Build history of the part. All positions in model axes, mm. Face numbers are marked on the shaded views. Round coordinates to 2 decimals unless told otherwise and drop trailing zeros. Write each loop counter-clockwise with the first axis right and the second up, starting at its lowest first coordinate (ties: lowest second). Pieces come first, ordered by that corner, then holes. Notation, with made-up numbers: (45.25, 29) - (73.25, 29) arc R16 cw to (73.25, 49) - close; hole circle Ø4 at (78.5, 3). An arc over 180 degrees is marked (long way). Answer as a JSON object with one key per item and string values. Group by question number.
Item 1: Slice it at C-C, the plane z = 5.25. List the corners of the cut face in (x, y), then the cut area to 3 significant figures.
Item 2: Probe line 1 (X direction, y = 0, z = 8); line 2 (X direction, y = 0, z = 6); line 3 (Y direction, x = -10, z = 11.25). List the from-to ranges inside material, lowest first. Write a range as from..to.
Item 3: Flat gauge pins, fed straight in: pin 1 (8 mm diameter, centred on x = -12.5, z = 2, fed in from +Y); pin 2 (3 mm diameter, centred on y = -10, z = 5.5, fed in from +X); pin 3 (10 mm diameter, centred on y = -16.5, z = 5.5, fed in from +X). Where does each tip first touch, or does it go through?
Item 4: Two-plate mould, pull along Y, no slides. Class the marked faces 1, 2 and 3: +Y half, -Y half, draft (parallel to the pull), parting line (faces both ways), or undercut.
Item 5: Slice it at D-D, the plane z = 10.5. List the corners of the cut face in (x, y), then the cut area to 3 significant figures.
Item 6: Slice it at A-A, the plane x = 0. List the corners of the cut face in (y, z).
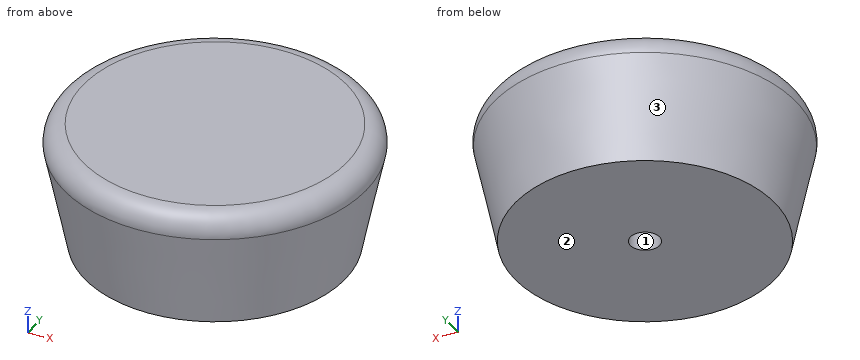
from build123d import *

# Parameters (mm, degrees)
F2_R     = 3
F3_R     = 2.25
F4_DEPTH = 16


with BuildPart() as f1:
    # F0 (on Front) → F1 (revolve)
    with BuildSketch(Plane.XZ):
        Polygon((0, 19), (0, 0), (20, 0), (24, 19), align=None)
    revolve(axis=Axis((0, 0, 9.5), (0, 0, 1)))

    # F2
    f2_edges = [f1.edges().sort_by_distance(p)[0] for p in [
        (-24, 0, 19),
    ]]
    fillet(f2_edges, radius=F2_R)

    # F3 (on face) → F4 (cut)
    with BuildSketch(Plane(origin=(0, 0, 0), x_dir=(1, 0, 0), z_dir=(0, 0, -1))):
        Circle(F3_R)
    extrude(amount=-F4_DEPTH, mode=Mode.SUBTRACT)


solid = f1.part
Geometry says:
{
 "1": {"outline": "circle Ø42.21 at (0, 0); hole circle Ø4.5 at (0, 0)", "area": "1,380 mm^2"},
 "2": {"line 1": "x = -21.68..-2.25, 2.25..21.68", "line 2": "x = -21.26..-2.25, 2.25..21.26", "line 3": "y = -20.01..20.01"},
 "3": {"pin 1": "stops at y = 18.79", "pin 2": "stops at x = 19.46", "pin 3": "stops at x = 17.99"},
 "4": {"face 1": "undercut", "face 2": "draft", "face 3": "parting line"},
 "5": {"outline": "circle Ø44.42 at (0, 0); hole circle Ø4.5 at (0, 0)", "area": "1,530 mm^2"},
 "6": {"outline": "(-23.24, 15.38) - (-20, 0) - (-2.25, 0) - (-2.25, 16) - (2.25, 16) - (2.25, 0) - (20, 0) - (23.24, 15.38) arc R3 ccw to (20.3, 19) - (-20.3, 19) arc R3 ccw to start"}
}
